from build123d import *


# Read off the part's stored shape, not the designer's step: Ø4.0mm 暗销孔1
with BuildPart() as part:
    # 草图1 → 旋转1 (revolve)
    with BuildSketch(Plane.XY, mode=Mode.PRIVATE) as revolve_1_sk:
        with BuildLine():
            Line((0, 17.25), (0, 24))
            Line((0, 24), (15, 24))
            Line((15, 24), (15, 35))
            Line((15, 35), (23, 35))
            Line((23, 35), (23, 20.66397832))
            ThreePointArc((23, 20.66397832), (28.202484376, 10.908712115), (30, 0))
            Line((30, 0), (24, 0))
            ThreePointArc((24, 0), (22.472147517, 9.122795944), (18.055328154, 17.25))
            Line((18.055328154, 17.25), (0, 17.25))
        make_face()
    revolve(revolve_1_sk.sketch.rotate(Axis((0, 0, 0), (1, 0, 0)), 90), axis=Axis((0, 0, 0), (1, 0, 0)))

    # Ø4.0mm 暗销孔1 outline → Ø4.0mm 暗销孔1 (revolve, cut)
    with BuildSketch(Plane(origin=(0, 29, 0), x_dir=(0, 1, 0), z_dir=(0, 0, -1))):
        Polygon((0, 23), (0, 18), (2, 19.201721238), (2, 23), align=None)
    revolve(axis=Axis((0, 29, 0), (1, 0, 0)), mode=Mode.SUBTRACT)

    # 4.0mm _1 2 outline → 4.0mm _1 2 (revolve, cut)
    with BuildSketch(Plane.YX.offset(-29)):
        Polygon((0, 23), (0, 18), (2, 19.201721238), (2, 23), align=None)
    revolve(axis=Axis((0, 0, 29), (1, 0, 0)), mode=Mode.SUBTRACT)

    # 4.0mm _1 3 outline → 4.0mm _1 3 (revolve, cut)
    with BuildSketch(Plane(origin=(0, -29, 0), x_dir=(0, 1, 0), z_dir=(0, 0, -1))):
        Polygon((0, 23), (0, 18), (2, 19.201721238), (2, 23), align=None)
    revolve(axis=Axis((0, -29, 0), (1, 0, 0)), mode=Mode.SUBTRACT)

    # 4.0mm _1 4 outline → 4.0mm _1 4 (revolve, cut)
    with BuildSketch(Plane.YX.offset(29)):
        Polygon((0, 23), (0, 18), (2, 19.201721238), (2, 23), align=None)
    revolve(axis=Axis((0, 0, -29), (1, 0, 0)), mode=Mode.SUBTRACT)


solid = part.part
Read the model definition and answer for the solid it produces. Units are mm, in the model's axes. A direction names the side the tool comes from. Give positions to 0.01 mm unless a question says otherwise; leave off trailing zeros. Write each loop counter-clockwise with the first axis right and the second up, starting at its lowest first coordinate (ties: lowest second). Pieces come first, ordered by that corner, then holes. Notation, with made-up numbers: (1.5, 36) - (7.5, 36) arc R22 cw to (7.5, 74) - close; hole circle Ø5 at (85.25, -0.5). An arc over 180 degrees is marked (long way). Answer in a Markdown table with one row per item. Add a question column.
Item 1: Section B-B, the plane y = 22.5 is taken. Write down the section's boundary in (x, z).
Item 2: Section D-D, the plane x = 26 is taken. Write down the section's boundary in (y, z).
Item 3: Section A-A, the plane x = 9 is taken. Write down the section's boundary in (y, z).
Item 4: Determine the mould class of faces 4 (the face through (18, 0, 29)), 5 (the face through (15, 23, 8)), 6 (the face through (19.056, 34.168, -7.587)) for opening direction Z: pulls with the +Z half, pulls with the -Z half, needs draft (parallel to the pull), parting line crosses it, or undercut.
Item 5: Section C-C, the plane z = 22 is taken. Write down the section's boundary in (x, y), and give its area (3 significant figures).
Item 6: Find the intervals of material crossed by L1, parallel to X at y = 27, z = -14.5; L2, parallel to Z at x = 4, y = -13.5; L3, parallel to Z at x = 20.4, y = -29, in increasing order.
Item 7: A tool of negligible diameter and unlimited length cuts with its end or side. For faces 1 (the face through (8.901, -0.758, -17.233)), 2 (the face through (0, 16, -10)), 3 (the face through (21, 0, -31)), from which of +Z, -Z, +X, -X, +Y, -Y can it reach the whole face along a straight path? Write none if from no direction.
Item 8: Flat-ended cylindrical pins translate along their axes: P1, Ø5, axis at y = 0, z = 29, coming from the +X side; P2, Ø3, axis at y = -29, z = 0, coming from the -X side; P3, Ø3, axis at y = 0, z = -29, coming from the +X side. Find the tip coordinate at first contact, or state that the pin passes through.
Recorded:
| question | item | result |
|---|---|---|
| 1 | outline | (0, -8.35) - (15, -8.35) - (15, -26.81) - (23, -26.81) - (23, 26.81) - (15, 26.81) - (15, 8.35) - (0, 8.35) - close |
| 2 | outline | circle Ø32 at (0, 0) |
| 3 | outline | circle Ø48 at (0, 0); hole circle Ø34.5 at (0, 0) |
| 4 | face 4 | undercut |
| 4 | face 5 | needs draft |
| 4 | face 6 | parting line crosses it |
| 5 | outline | (0, -9.59) - (15, -9.59) - (15, -27.22) - (23, -27.22) - (23, 27.22) - (15, 27.22) - (15, 9.59) - (0, 9.59) - close |
| 5 | area | 723 mm2 |
| 6 | L1 | x = 15 to 23 |
| 6 | L2 | z = -19.84 to -10.74, 10.74 to 19.84 |
| 6 | L3 | z = -19.6 to -2, 2 to 19.6 |
| 7 | face 1 | -X |
| 7 | face 2 | +Z, -Z, -X, +Y, -Y |
| 7 | face 3 | +X |
| 8 | P1 | stops at x = 23 |
| 8 | P2 | stops at x = 15 |
| 8 | P3 | stops at x = 18.9 |
